Source: three-view drawing plus pictorial views. Frame: mm from the lowest corner of the part. A direction names the side the tool comes from. Give positions to 0.01 mm unless a question says otherwise; leave off trailing zeros. Loops run counter-clockwise (first coordinate to the right, second up) from the corner with the lowest first, then second, coordinate; pieces in that order, holes last. Notation, with made-up numbers: (-35.5, 41.25) - (-16.5, 41.25) arc R13 cw to (-16.5, 61.25) - close; hole circle Ø5 at (77.5, 53.5). An arc over 180 degrees is marked (long way). Answer as a JSON object with one key per item and string values.
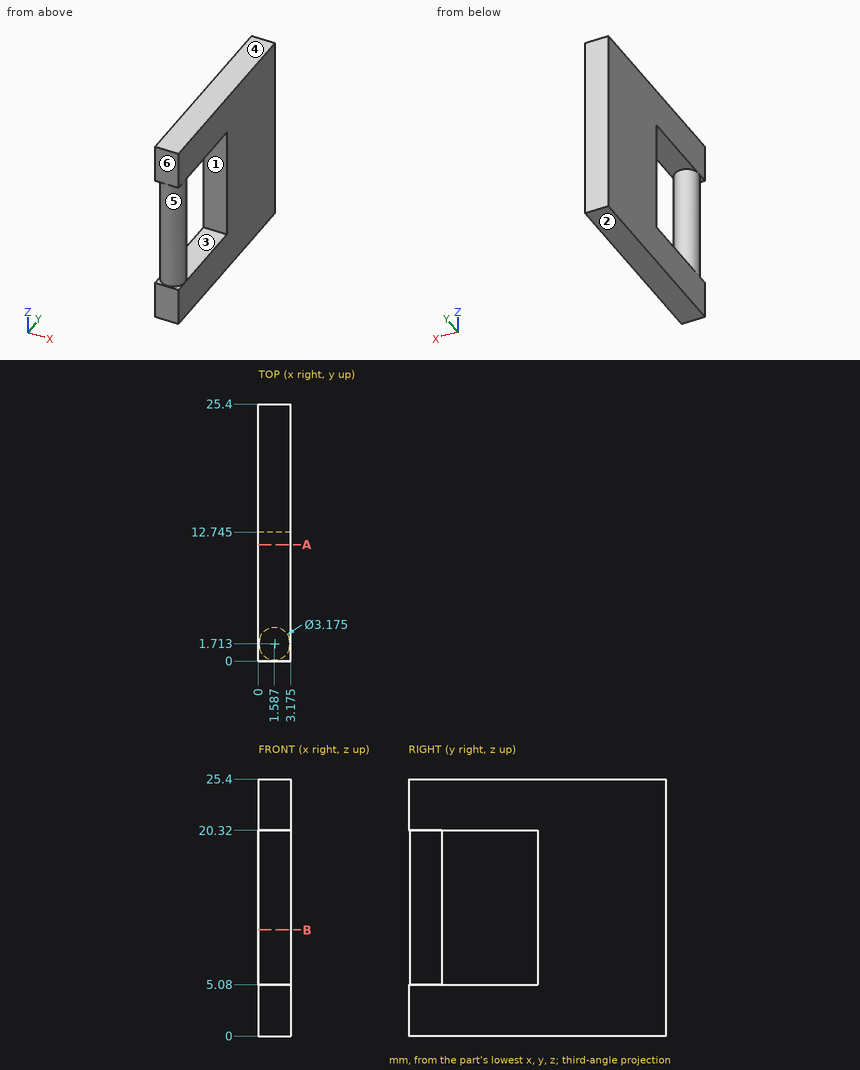
Item 1: Access query for the marked faces 5 and 6. Directions: +Z, -Z, +X, -X, +Y, -Y. A direction counts if a zero-diameter tool reaches every point of the face in a straight line with its end or side. Return the directions, or none.
Geometry check:
{"face 5": "none", "face 6": "+Z, -Z, +X, -X, -Y"}
Item 2: Cut plane B-B (z = 10.5). Return loops of the section in (x, y) (1 decimal), then the cut area to 3 significant figures.
Geometry check:
{"outline": "circle Ø3.2 at (1.6, 1.7); (0, 12.7) - (3.2, 12.7) - (3.2, 25.4) - (0, 25.4) - close", "area": "48.1 mm2"}
Item 3: Cut plane A-A (y = 11.5). Return loops of the section in (x, z) (1 decimal).
Geometry check:
{"outline": "(0, 0) - (3.2, 0) - (3.2, 5.1) - (0, 5.1) - close; (0, 20.3) - (3.2, 20.3) - (3.2, 25.4) - (0, 25.4) - close"}
Item 4: Mould query, pull axis Z, two halves, no side actions, for the marked faces 1, 2, 3 and 4. Classes: released by +Z, released by -Z, zero draft, split by the parting line, or undercut.
Geometry check:
{"face 1": "undercut", "face 2": "released by -Z", "face 3": "undercut", "face 4": "released by +Z"}
Item 5: Material intervals for line 1 (Z direction, x = 2.85, y = 8); line 2 (Y direction, x = 0.9, z = 19) (1 decimal); line 3 (Y direction, x = 2.65, z = 9) (1 decimal), sorted ascending. Write a range as [from, to].
Geometry check:
{"line 1": "z = [0, 5.08], [20.32, 25.4]", "line 2": "y = [0.3, 3.1], [12.7, 25.4]", "line 3": "y = [0.5, 2.9], [12.7, 25.4]"}
Item 6: Contact query for a flat-ended pin moving along its axis: P1, Ø1.6, axis at x = 1.5, z = 9.5, coming from the -Y side (1 decimal). Output: stop coordinate, or through.
Geometry check:
{"P1": "stops at y = 0.1"}
